Here's how the part is built. I have some questions about the finished solid (model axes, mm). Face numbers are marked on the shaded views. A direction names the side the tool comes from. Round coordinates to 2 decimals unless told otherwise and drop trailing zeros. Loops run counter-clockwise (first coordinate to the right, second up) from the corner with the lowest first, then second, coordinate; pieces in that order, holes last. Notation, with made-up numbers: M 59.5,68 L 68.5,68 A26 ccw 68.5,104 Z; hole C -26,64.25 d11. An arc over 180 degrees is marked long. Use a Markdown table: item, result.
```python
from build123d import *

# Parameters (mm, degrees)
CROQUIS2_W              = 13.8
CROQUIS2_H              = 10
SALIENTE_EXTRUIR1_DEPTH = 2.2
CROQUIS3_W              = 11.8
CROQUIS3_H              = 8
SALIENTE_EXTRUIR2_DEPTH = 6.3
CROQUIS4_R              = 3.5
CORTAR_EXTRUIR1_DEPTH   = 8


with BuildPart() as part:
    # Croquis2 → Saliente-Extruir1 (new body)
    with BuildSketch(Plane(origin=(0, 0, 0), x_dir=(1, 0, 0), z_dir=(0, 1, 0))):
        with Locations((-0.655307263, 0.782122905)):
            Rectangle(CROQUIS2_W, CROQUIS2_H)
    extrude(amount=SALIENTE_EXTRUIR1_DEPTH)

    # Croquis3 → Saliente-Extruir2 (add)
    with BuildSketch(Plane(origin=(0, 2.2, 0), x_dir=(1, 0, 0), z_dir=(0, 1, 0))):
        with Locations((-0.655307263, 0.782122905)):
            Rectangle(CROQUIS3_W, CROQUIS3_H)
    extrude(amount=SALIENTE_EXTRUIR2_DEPTH)

    # Croquis4 → Cortar-Extruir1 (cut)
    with BuildSketch(Plane.XZ):
        with Locations((-0.655307263, -0.782122905)):
            Circle(CROQUIS4_R)
    extrude(amount=-CORTAR_EXTRUIR1_DEPTH, mode=Mode.SUBTRACT)


solid = part.part
```
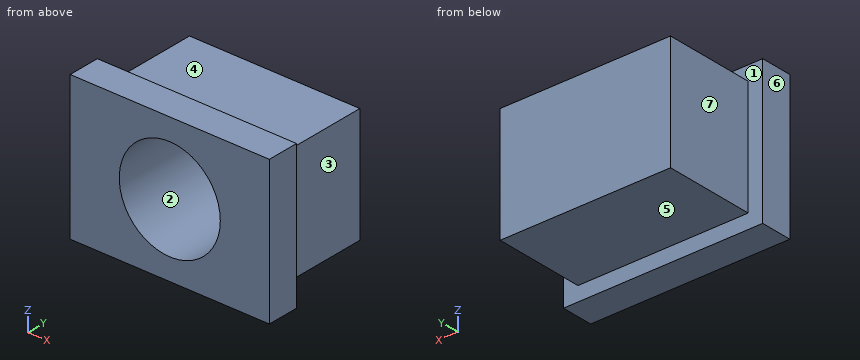
Q1. For the marked faces 4, 5, 6 and 7, which set-ups out of +Z, -Z, +X, -X, +Y, -Y let a thin tool reach every point of the face, with its end or its side?
Return value:
| item | result |
|---|---|
| face 4 | +Z, +X, -X, +Y |
| face 5 | -Z, +X, -X, +Y |
| face 6 | +Z, -Z, -X, +Y, -Y |
| face 7 | +Z, -Z, -X, +Y |
Q2. Will these pins go through, and if not, where does the flat tip stop? P1, Ø3, axis at x = -3, y = 4, coming from the -Z side; P2, Ø2, axis at x = 1, z = -0.5, coming from the -Y side; P3, Ø1.9, axis at x = -0.5, y = 6.5, coming from the +Z side; P4, Ø1.5, axis at y = 2.5, z = -3.5, coming from the -X side.
Return value:
| item | result |
|---|---|
| P1 | stops at z = -4.78 |
| P2 | stops at y = 8 |
| P3 | stops at z = 3.22 |
| P4 | stops at x = -7.56 |
Q3. Imagine slicing it at B-B, the plane y = 6. Please give me the cut outline in (x, z), then the cut area to 3 significant figures.
Return value:
| item | result |
|---|---|
| outline | M -6.56,-4.78 L 5.24,-4.78 L 5.24,3.22 L -6.56,3.22 Z; hole C -0.66,-0.78 d7 |
| area | 55.9 mm^2 |
Q4. I need wall thicknesses on line 1 (Z direction, x = -4.5, y = 6.5); line 2 (Y direction, x = 1.5, z = -1); line 3 (Y direction, x = -6.75, z = -1.5). Which ranges of each line are inside material? Lowest first, please. Write a range as from..to.
Return value:
| item | result |
|---|---|
| line 1 | z = -4.78..3.22 |
| line 2 | y = 8..8.5 |
| line 3 | y = 0..2.2 |
Q5. We'd pull the mould along X, two halves only. Please class the marked faces 1, 2 and 3: pulls with the +X half, pulls with the -X half, needs draft (parallel to the pull), parting line crosses it, or undercut.
Return value:
| item | result |
|---|---|
| face 1 | needs draft |
| face 2 | undercut |
| face 3 | pulls with the +X half |
Q6. Imagine slicing it at A-A, the plane x = -6.25. Please give me the cut outline in (y, z).
Return value:
| item | result |
|---|---|
| outline | M 0,-5.78 L 2.2,-5.78 L 2.2,-4.78 L 8.5,-4.78 L 8.5,3.22 L 2.2,3.22 L 2.2,4.22 L 0,4.22 Z |
Q7. Imagine slicing it at C-C, the plane z = 1.75. Please give me the cut outline in (x, y).
Return value:
| item | result |
|---|---|
| outline | M -7.56,0 L -3.07,0 L -3.07,8 L 1.76,8 L 1.76,0 L 6.24,0 L 6.24,2.2 L 5.24,2.2 L 5.24,8.5 L -6.56,8.5 L -6.56,2.2 L -7.56,2.2 Z |
Q8. Imagine slicing it at D-D, the plane y = 1.5. Please give me the cut outline in (x, z), then the cut area to 3 significant figures.
Return value:
| item | result |
|---|---|
| outline | M -7.56,-5.78 L 6.24,-5.78 L 6.24,4.22 L -7.56,4.22 Z; hole C -0.66,-0.78 d7 |
| area | 99.5 mm^2 |
